The listing builds one solid part. Answer for the finished solid, in the listing's coordinates (mm). A direction names the side the tool comes from. Round coordinates to 2 decimals unless told otherwise and drop trailing zeros. Write each loop counter-clockwise with the first axis right and the second up, starting at its lowest first coordinate (ties: lowest second). Pieces come first, ordered by that corner, then holes. Notation, with made-up numbers: M 61,36.25 L 73,36.25 A20 ccw 73,59.25 Z; hole C -39.5,59 d2. An arc over 180 degrees is marked long. Write each question's results on one line, items separated by ' | '.
from build123d import *

# Parameters (mm, degrees)
F0_R            = 2.15265
F0_R_2          = 3.96875
F0_W            = 7.874
F0_H            = 3.175
F1_DEPTH        = 10.795
F2_R            = 1.8288
F3_REACH        = 42.4798775257
F5_R            = 3.96875
F6_DEPTH        = 4.445
F8_DEPTH        = 10.795
F8_COPIES_COUNT = 3
F8_COPIES_ANGLE = 180
F9_R            = 0.762
F11_R           = 3.96875
F11_R_2         = 2.15265
F13_DEPTH       = 6.35


# Not quite as in the source:
# - a feature of the source that left no trace in its solid (it failed there, or was rolled back) is left out
# - a pattern or mirror of a feature is missing from the dataset's text; its kind, count and spacing are read off the source's solid


with BuildPart() as f1:
    # F0 (on Top) → F1 (new body)
    with BuildSketch(Plane.XY):
        with BuildLine():
            Line((3.96875, 15.08125), (-3.96875, 15.08125))
            Line((-3.96875, 15.08125), (-3.96875, 21.8677764859))
            ThreePointArc((-3.96875, 21.8677764859), (0, -22.225), (3.96875, 21.8677764859))
            Line((3.96875, 21.8677764859), (3.96875, 15.08125))
        make_face()
        with Locations((-11.7865861589, -11.7865861589)):
            Circle(F0_R, mode=Mode.SUBTRACT)
        with Locations((11.7865861589, -11.7865861589)):
            Circle(F0_R, mode=Mode.SUBTRACT)
        with Locations((-11.7865861589, 11.7865861589)):
            Circle(F0_R, mode=Mode.SUBTRACT)
        Circle(F0_R_2, mode=Mode.SUBTRACT)
        with Locations((0, 8.73125)):
            Rectangle(F0_W, F0_H, mode=Mode.SUBTRACT)
        with Locations((11.7865861589, 11.7865861589)):
            Circle(F0_R, mode=Mode.SUBTRACT)
    extrude(amount=F1_DEPTH)

    f3_end = f1.faces().sort_by_distance((-3.96875, 0, 5.3975))[0]
    # F2 (on face) → F3 (cut, up to a face of the model that its end follows)
    with BuildSketch(Plane(origin=(0, 15.08125, 0), x_dir=(-1, 0, 0), z_dir=(0, 1, 0))):
        with Locations((0, 5.3975)):
            Circle(F2_R)
    f3_long = extrude(amount=-F3_REACH, mode=Mode.PRIVATE)
    add(split(f3_long, bisect_by=f3_end, keep=Keep.ALL, mode=Mode.PRIVATE).solids().sort_by_distance((0, 15.08125, 5.3975))[0], mode=Mode.SUBTRACT)

    # F5 (on face) → F6 (cut, through all)
    with BuildSketch(Plane(origin=(0, 0, 0), x_dir=(1, 0, 0), z_dir=(0, 0, -1))):
        with Locations((11.7865861589, -11.7865861589)):
            Circle(F5_R)
        with Locations((-11.7865861589, 11.7865861589)):
            Circle(F5_R)
    extrude(amount=-F6_DEPTH, mode=Mode.SUBTRACT)

    # F7 (on face) → F8 (cut, through all)
    with BuildSketch(Plane(origin=(0, 0, 0), x_dir=(1, 0, 0), z_dir=(0, 0, -1))):
        with BuildLine():
            ThreePointArc((-17.3148424047, -11.229543123), (-14.7565267097, -7.0906978311), (-9.9206262673, -6.5530302219))
            Line((-9.9206262673, -6.5530302219), (-6.4462980227, -3.0787019773))
            ThreePointArc((-6.4462980227, -3.0787019773), (-7.14375, 0), (-6.4462980227, 3.0787019773))
            Line((-6.4462980227, 3.0787019773), (-9.9206262673, 6.5530302219))
            ThreePointArc((-9.9206262673, 6.5530302219), (-14.7565267097, 7.0906978311), (-17.3148424047, 11.229543123))
            ThreePointArc((-17.3148424047, 11.229543123), (-20.6375, 0), (-17.3148424047, -11.229543123))
        make_face()
    f8 = extrude(amount=-F8_DEPTH, mode=Mode.SUBTRACT)

    # F8_copies: F8 ×3 about axis
    f8_copies_axis = Axis((0, 0, 0), (0, 0, 1))
    for i in range(1, F8_COPIES_COUNT):
        add(f8.rotate(f8_copies_axis, i * F8_COPIES_ANGLE / (F8_COPIES_COUNT - 1)), mode=Mode.SUBTRACT)

    # F9
    f9_edges = [f1.edges().sort_by_distance(p)[0] for p in [
        (-17.314842, -11.229543, 5.3975),
        (-9.920626, -6.55303, 5.3975),
        (-6.446298, -3.078702, 5.3975),
        (-6.446298, 3.078702, 5.3975),
        (-9.920626, 6.55303, 5.3975),
        (-17.314842, 11.229543, 5.3975),
        (3.96875, 21.867776, 5.3975),
        (-3.96875, 21.867776, 5.3975),
        (11.229543, -17.314842, 5.3975),
        (-11.229543, -17.314842, 5.3975),
        (6.55303, -9.920626, 5.3975),
        (-6.55303, -9.920626, 5.3975),
        (3.078702, -6.446298, 5.3975),
        (-3.078702, -6.446298, 5.3975),
        (17.314842, 11.229543, 5.3975),
        (17.314842, -11.229543, 5.3975),
        (9.920626, 6.55303, 5.3975),
        (6.446298, 3.078702, 5.3975),
        (6.446298, -3.078702, 5.3975),
        (9.920626, -6.55303, 5.3975),
    ]]
    fillet(f9_edges, radius=F9_R)

    # F11 (on face) → F13 (cut, through all)
    with BuildSketch(Plane.XY.offset(10.795)):
        with Locations((-11.7865861589, 11.7865861589)):
            Circle(F11_R)
        with Locations((-11.7865861589, 11.7865861589)):
            Circle(F11_R_2, mode=Mode.SUBTRACT)
        with Locations((11.7865861589, -11.7865861589)):
            Circle(F11_R)
        with Locations((11.7865861589, -11.7865861589)):
            Circle(F11_R_2, mode=Mode.SUBTRACT)
    extrude(amount=-F13_DEPTH, mode=Mode.SUBTRACT)


solid = f1.part
1) Section B-B (y = 0) is taken. Determine the outline of the cut face in (x, z) (1 decimal), then the cut area to 3 significant figures.
Return value:
outline: M -22.2,0 L -20.6,0 L -20.6,10.8 L -22.2,10.8 Z; M -7.1,0 L -4,0 L -4,10.8 L -7.1,10.8 Z; M 4,0 L 7.1,0 L 7.1,10.8 L 4,10.8 Z; M 20.6,0 L 22.2,0 L 22.2,10.8 L 20.6,10.8 Z | area: 103 mm²
2) Section A-A (x = 0) is taken. Determine the outline of the cut face in (y, z) (1 decimal).
Return value:
outline: M -22.2,0 L -20.6,0 L -20.6,10.8 L -22.2,10.8 Z; M -7.1,0 L -4,0 L -4,10.8 L -7.1,10.8 Z; M 4,0 L 7.1,0 L 7.1,3.6 L 4,3.6 Z; M 4,7.2 L 7.1,7.2 L 7.1,10.8 L 4,10.8 Z; M 10.3,0 L 15.1,0 L 15.1,3.6 L 10.3,3.6 Z; M 10.3,7.2 L 15.1,7.2 L 15.1,10.8 L 10.3,10.8 Z
3) Section C-C (y = 17) is taken. Determine the outline of the cut face in (x, z) (3 decimals).
Return value:
outline: M -14.316,0 L -3.969,0 L -3.969,10.795 L -14.316,10.795 Z; M 3.969,0 L 14.316,0 L 14.316,10.795 L 3.969,10.795 Z
4) Find the intervals of material crossed by line 1 (Z direction, x = 0, y = 13.25) (3 decimals); line 2 (Y direction, x = -8.5, z = 6); line 3 (Y direction, x = 9, z = 0.75), in increasing order.
Return value:
line 1: 0 to 3.569, 7.226 to 10.795 | line 2: -20.54 to -18.81, -16.27 to -5.13, 5.13 to 9.56, 14.01 to 20.54 | line 3: -20.32 to -18.57, -16.59 to -5.63, 5.63 to 8.96, 14.61 to 20.32
5) Each of these flat-tipped pins is pushed along its axis until it touches: pin 1 (2.5 mm diameter, centred on x = 11.79, y = -11.79, fed in from -Z); pin 2 (3 mm diameter, centred on x = -6.5, z = 2.5, fed in from -Y); pin 3 (4 mm diameter, centred on y = -16.5, z = 7.5, fed in from -X); pin 4 (3.5 mm diameter, centred on x = 0, z = 5.4, fed in from +Y). Where does it stop, or does it pass through?
Return value:
pin 1: through | pin 2: y = -21.66 | pin 3: x = -16.84 | pin 4: y = -3.56
6) A tool of negligible diameter and unlimited length cuts with its end or side. For faces 1 (the face through (15.45, -13.31, 7.66)), 2 (the face through (1.827, 5.358, 5.478)), 3 (the face through (6.755, -14.144, 5.322)), from which of +Z, -Z, +X, -X, +Y, -Y can it reach the whole face along a straight path? Write none if from no direction.
Return value:
face 1: +Z | face 2: +Y | face 3: +Z, -Z
7) Section D-D (z = 6.5) is taken. State how many separate pieces and enclosed holes the cut face has, then the cut area to 3 significant figures.
Return value:
separate pieces: 1 | enclosed holes: 7 | area: 714 mm²
8) The mould has two halves that part along Y. Classify faces 4 (the face through (0.396, 12.733, 3.612)), 5 (the face through (20.637, 0.14, 5.322)): +Y half, -Y half, draft (parallel to the pull), parting line (faces both ways), or undercut.
Return value:
face 4: draft | face 5: undercut
